Autodesk Fusion 360 part; units mm, degrees
ref_plane "WorkPlane3" through (50, 0, 0) normal (1, 0, 0) x (0, 1, 0) in component "Container"
sketch "Sketch6" plane through (0, 0, 0) normal (0, 1, 0) x (1, 0, 0) in component "Container"
  line L0 (0, 0) -> (55.25, 0)
  line L1 (55.25, 0) -> (55.25, -3)
  line L2 (55.25, -3) -> (0, -3)
  line L3 (0, -3) -> (0, 0)
  line L4 (50.25, -13) -> (55.25, -13)
  line L5 (55.25, -13) -> (55.25, -3)
  line L6 (55.25, -3) -> (50.25, -3)
  line L7 (50.25, -3) -> (50.25, -13)
  line L8 (50.25, -13) -> (104.5, -13) construction
  line L9 (50.25, -13) -> (47.7874, -16.152)
  line L10 (50.25, -13) -> (104.5, -13) construction
  line L11 (47.7874, -16.152) -> (55.25, -16.152)
  line L12 (55.25, -13) -> (55.25, -16.152)
  line L13 (50.25, -13) -> (50.25, -16.152) construction
  line L14 (50.25, -16.152) -> (55.25, -16.152)
  line L15 (55.25, -16.152) -> (55.25, -47.152)
  line L16 (55.25, -47.152) -> (50.25, -47.152)
  line L17 (50.25, -47.152) -> (50.25, -16.152)
  dimension "d44" = 55.25
  dimension "d45" = 3
  dimension "d47" = 10
  dimension "d48" = 10
  dimension "d49" = 5
  dimension "d50" = 5
  dimension "d53" = 128
  dimension "d54" = 4
  dimension "d56" = 3.152
  dimension "d57" = 5
  dimension "d58" = 31
revolve "Revolve1" add sketch "Sketch6" angle 360 about axis through (0, 0, 1.75) along (0, 0, 1) makes body 1 in component "Container"
fillet "Fillet2" radius 2 1 edges at (-51.5111, -19.9793, 47.152) on bodies 1 in component "Container"
copy_body "CutPasteBodies1" bodies 1 removing the originals makes body 2 in component "Container"
sketch "Sketch8" plane through (50, 0, 0) normal (1, 0, 0) x (0, 1, 0)
  line L0 (-5, 11) -> (5, 11)
  line L1 (5, 11) -> (5, 4)
  line L2 (5, 4) -> (-5, 4)
  line L3 (-5, 4) -> (-5, 11)
  dimension "d71" = 7
  dimension "d72" = 10
  dimension "d73" = 5
  dimension "d74" = 4
extrude "Extrude1" cut sketch "Sketch8" along normal blind 17 bodies 2 in component "Container"
fillet "Fillet1" radius 2 4 edges at (52.512, -5, 11) (52.512, 5, 11) (52.512, -5, 4) (52.512, 5, 4) on bodies 2 in component "Container"
component "Container" placed x (1, 0, 0) y (0, 1, 0) z (0, 0, 1) at (0, 0, 0)
equation "d44 = ( 100.5 / 2 ) * 1 mm + d49"
equation "d48 = d47"
equation "d50 = d49"
equation "d53 = 90 deg + 38 deg"
equation "d57 = d49"
equation "d73 = d72 / 2"
equation "d74 = 3.00 mm + 1 mm"
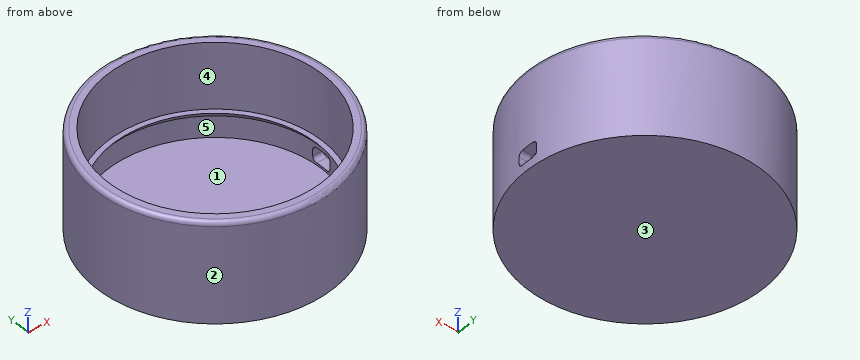
Verification items for the finished model (mm, model axes). Face numbers are marked on the shaded views. A direction names the side the tool comes from. Round coordinates to 2 decimals unless told otherwise and drop trailing zeros. Order: outer loops, then holes, each group sorted by start corner. A loop starts at its lowest first (then second) coordinate and runs counter-clockwise, first axis right, second up.
1. Release check for a two-part mould opening along Y. For the marked faces 1, 2 and 3 record: +Y half, -Y half, draft (parallel to the pull), parting line (faces both ways), or undercut.
Final values:
face 1: undercut
face 2: parting line
face 3: draft
2. Section check B-B on y = 0. Record the cut outline in (x, z), then the cut area to 3 significant figures.
Final values:
outline: (-55.25, 0) - (55.25, 0) - (55.25, 4) - (50.25, 4) - (50.25, 3) - (-50.25, 3) - (-50.25, 13) - (-47.79, 16.15) - (-50.25, 16.15) - (-50.25, 47.15) - (-53.25, 47.15) arc R2 ccw to (-55.25, 45.15) - close; (47.79, 16.15) - (50.25, 13) - (50.25, 11) - (55.25, 11) - (55.25, 45.15) arc R2 ccw to (53.25, 47.15) - (50.25, 47.15) - (50.25, 16.15) - close
area: 744 mm2
3. Section check C-C on x = 0. Record the cut outline in (y, z).
Final values:
outline: (-55.25, 0) - (55.25, 0) - (55.25, 45.15) arc R2 ccw to (53.25, 47.15) - (50.25, 47.15) - (50.25, 16.15) - (47.79, 16.15) - (50.25, 13) - (50.25, 3) - (-50.25, 3) - (-50.25, 13) - (-47.79, 16.15) - (-50.25, 16.15) - (-50.25, 47.15) - (-53.25, 47.15) arc R2 ccw to (-55.25, 45.15) - close
4. Go/stop test with flat-tipped pins: P1, Ø3.5, axis at x = 53, z = 8, coming from the +Y side; P2, Ø3, axis at x = 10.5, z = 18, coming from the -Y side; P3, Ø6, axis at x = -22, z = 31.5, coming from the -Y side. Record where each tip stops, or that it passes through.
Final values:
P1: stops at y = 20.64
P2: stops at y = -54.51
P3: stops at y = -51.88
5. Section check A-A on z = 32.5. Record the cut outline in (x, y), then the cut area to 3 significant figures.
Final values:
outline: circle Ø110.5 at (0, 0); hole circle Ø100.5 at (0, 0)
area: 1,660 mm2
6. Thickness scan on L1, parallel to Y at x = 0, z = 36; L2, parallel to Z at x = 22, y = 33.5; L3, parallel to X at y = 26.5, z = 45. Record the ranges inside material, lowest first.
Final values:
L1: y = -55.25 to -50.25, 50.25 to 55.25
L2: z = 0 to 3
L3: x = -48.48 to -42.69, 42.69 to 48.48
7. Access from +Z, -Z, +X, -X, +Y, -Y to the whole of each face (thin tool, end or side, straight path). Record for the marked faces 4 and 5.
Final values:
face 4: +Z
face 5: none
